For this review, take the finished solid that the model builds, in its own axes (mm). Face numbers are marked on the shaded views. A direction names the side the tool comes from. Coordinates: 2 decimals unless noted, no trailing zeros. Loops run counter-clockwise (first coordinate to the right, second up) from the corner with the lowest first, then second, coordinate; pieces in that order, holes last. Notation, with made-up numbers: M 1,-32 L 41,-32 A30 cw 41,3 Z; hole C -26.75,25 d7. An arc over 180 degrees is marked long. Put each result on its own line as item: value.
```python
from build123d import *

# Parameters (mm, degrees)
SKETCH3_R           = 2
BOSS_EXTRUDE1_DEPTH = 1


with BuildPart() as part:
    # Sketch1 → Revolve1 (revolve)
    with BuildSketch(Plane(origin=(0, 0, 0), x_dir=(1, 0, 0), z_dir=(0, 1, 0))):
        with BuildLine():
            Line((0, 8.5), (0, -8.5))
            ThreePointArc((0, -8.5), (8.5, 0), (0, 8.5))
        make_face()
    revolve(axis=Axis((0, 0, -8.5), (0, 0, 1)))

    # Sketch2 → Revolve2 (revolve)
    with BuildSketch(Plane.XY, mode=Mode.PRIVATE) as revolve2_sk:
        with BuildLine():
            Line((13, 6.618380291), (13, 11))
            Line((13, 11), (0, 11))
            Line((0, 11), (0, 10))
            Line((0, 10), (12, 10))
            Line((12, 10), (12, 6.618380291))
            ThreePointArc((12, 6.618380291), (11.018242025, 1.864608874), (8.233609553, -2.111320376))
            ThreePointArc((8.233609553, -2.111320376), (7.923281837, -3.077597265), (7.5, -4))
            ThreePointArc((7.5, -4), (11.543396381, 0.639249919), (13, 6.618380291))
        make_face()
    revolve(revolve2_sk.sketch.rotate(Axis((0, 11, 0), (0, -1, 0)), 90), axis=Axis((0, 11, 0), (0, -1, 0)))

    # Sketch3 → Boss-Extrude1 (add)
    with BuildSketch(Plane(origin=(0, 11, 0), x_dir=(1, 0, 0), z_dir=(0, 1, 0))):
        with BuildLine():
            Line((-21.894736842, 4.076824575), (-9.263157895, 13.04583864))
            ThreePointArc((-9.263157895, 13.04583864), (0, 16), (9.263157895, 13.04583864))
            Line((9.263157895, 13.04583864), (21.894736842, 4.076824575))
            ThreePointArc((21.894736842, 4.076824575), (24, 0), (21.894736842, -4.076824575))
            Line((21.894736842, -4.076824575), (9.263157895, -13.04583864))
            ThreePointArc((9.263157895, -13.04583864), (0, -16), (-9.263157895, -13.04583864))
            Line((-9.263157895, -13.04583864), (-21.894736842, -4.076824575))
            ThreePointArc((-21.894736842, -4.076824575), (-24, 0), (-21.894736842, 4.076824575))
        make_face()
        with Locations(Location((-19, 0, 0), (0, 0, 270))):
            Circle(SKETCH3_R, mode=Mode.SUBTRACT)
        with Locations(Location((19, 0, 0), (0, 0, 90))):
            Circle(SKETCH3_R, mode=Mode.SUBTRACT)
    extrude(amount=BOSS_EXTRUDE1_DEPTH)


solid = part.part
```
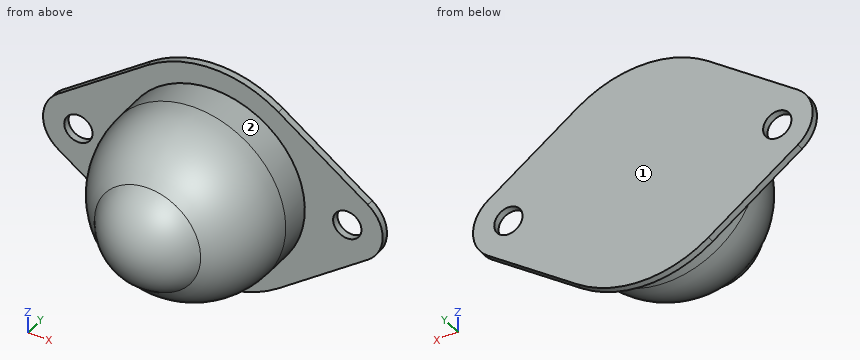
(1) For pin 1 (1 mm diameter, centred on x = 4.5, y = -4.5, fed in from +Z); pin 2 (3 mm diameter, centred on x = 14.5, z = 4, fed in from -Y); pin 3 (5 mm diameter, centred on x = -4, z = -11, fed in from -Y), all flat-tipped, find the tip position at first contact; note any pin that passes through.
Determined:
pin 1: stops at z = 6.15
pin 2: stops at y = 11
pin 3: stops at y = -2.56
(2) Add section B-B (z = 0). Write out the cut boundary in (x, y).
Determined:
outline: M -24,11 L -21,11 L -21,12 L -24,12 Z; M -17,11 L -13,11 L -13,6.62 A13 ccw -7.5,-4 A8.5 ccw 7.5,-4 A13 ccw 13,6.62 L 13,11 L 17,11 L 17,12 L -17,12 Z; M 21,11 L 24,11 L 24,12 L 21,12 Z; hole M -12,6.62 A12 ccw -8.23,-2.11 A8.5 cw long 8.23,-2.11 A12 ccw 12,6.62 L 12,10 L -12,10 Z
(3) Add section A-A (x = -18.5). Write out the cut boundary in (y, z), plus the area to 3 significant figures.
Determined:
outline: M 11,-6.49 L 12,-6.49 L 12,-1.94 L 11,-1.94 Z; M 11,1.94 L 12,1.94 L 12,6.49 L 11,6.49 Z
area: 9.10 mm^2
(4) Add section D-D (x = 4). Write out the cut boundary in (y, z), plus the area to 3 significant figures.
Determined:
outline: M -4,-6.34 A12.37 ccw 6.62,-12.37 L 11,-12.37 L 11,-15.49 L 12,-15.49 L 12,15.49 L 11,15.49 L 11,12.37 L 6.62,12.37 A12.37 ccw -4,6.34 A7.5 ccw Z; hole M -2.11,-7.2 A11.31 ccw 6.62,-11.31 L 10,-11.31 L 10,11.31 L 6.62,11.31 A11.31 ccw -2.11,7.2 A7.5 cw long Z
area: 263 mm^2
(5) Add section C-C (y = 1.75). Write out the cut boundary in (x, z), plus the area to 3 significant figures.
Determined:
outline: C 0,0 d24.11; C 0,0 d16.64; hole C 0,0 d21.94
area: 296 mm^2
(6) Wall thickness on line 1 along X through (y, z) = (11.35, 0); line 2 along X through (y, z) = (5.25, 3.5); line 3 along Y through (x, z) = (0.5, -7): over which ranges is each line inside the solid? List them lowest first. Write a range as [from, to].
Determined:
line 1: x = [-24, -21], [-17, 17], [21, 24]
line 2: x = [-12.44, -11.4], [-5.7, 5.7], [11.4, 12.44]
line 3: y = [-4.8, 4.8], [10, 12]
(7) Tool access review of the marked faces 1 and 2: name each direction out of +Z, -Z, +X, -X, +Y, -Y from which nothing blocks a thin tool from reaching the whole face with its end or side.
Determined:
face 1: +Z, -Z, +X, -X, +Y
face 2: -Y
